Design review of the part built by this model. Coordinates are the model's own, in mm. A direction names the side the tool comes from. Coordinates: 2 decimals unless noted, no trailing zeros. Loops run counter-clockwise (first coordinate to the right, second up) from the corner with the lowest first, then second, coordinate; pieces in that order, holes last.
Autodesk Inventor part; units mm, degrees
ref_plane "YZ Plane" through (0, 0, 0) normal (1, 0, 0) x (0, 1, 0)
ref_plane "XZ Plane" through (0, 0, 0) normal (0, 1, 0) x (-1, 0, 0)
ref_plane "XY Plane" through (0, 0, 0) normal (0, 0, 1) x (1, 0, 0)
sketch "Sketch1" plane through (0, 0, 0) normal (0, 1, 0) x (-1, 0, 0)
  circle A0 centre (0, 0) radius 43.5
  dimension "d0" = 87
extrude "Extrusion1" add sketch "Sketch1" along normal blind 13
sketch "Sketch2" plane through (0, 13, 0) normal (0, 1, 0) x (1, 0, 0)
  circle A0 centre (0, 0) radius 43.5
  line L0 (0, 55.4914) -> (0, 55.5)
  circle A1 centre (0, 0) radius 43.5
  line L1 (43.5, 0) -> (43.5, 37)
  line L2 (0, 55.5) -> (1, 55.5)
  line L3 (1, 55.5) -> (1, 43.5)
  line L4 (0, 55.4914) -> (0, 55.5)
  arc A2 (43.5, 37) -> (1, 55.5) centre (1, -2.5676) ccw
  line L5 (1, 43.4885) -> (1, 43.5)
  line L6 (-55.5, 1) -> (-43.5, 1)
  arc A3 (-37, 43.5) -> (-55.5, 1) centre (2.5676, 1) ccw
  line L7 (0, 43.5) -> (-37, 43.5)
  line L8 (-1, -55.5) -> (-1, -43.5)
  arc A4 (-43.5, -37) -> (-1, -55.5) centre (-1, 2.5676) ccw
  line L9 (-43.5, 0) -> (-43.5, -37)
  line L10 (55.5, -1) -> (43.5, -1)
  arc A5 (37, -43.5) -> (55.5, -1) centre (-2.5676, -1) ccw
  line L11 (0, -43.5) -> (37, -43.5)
  point P0 (0, 43.5)
  point P1 (43.5, 0)
  point P2 (-55.4914, 0)
  point P3 (0, -55.4914)
  point P4 (55.4914, 0)
  dimension "d3" = 12
  dimension "d75" = 1
  dimension "d91" = 37
  dimension "d92" = 58.0676
  dimension "d93" = 42.5
  dimension "d94" = 0
  dimension "d95" = 87.5
  dimension "d110" = 360
extrude "Extrusion2" add sketch "Sketch2" against normal blind 13 contours A0 L5 L3 A2 L1
sketch "Sketch6" plane through (0, 0, 0) normal (0, -1, 0) x (1, 0, 0)
  circle A0 centre (0, 0) radius 43.5
  point P0 (0, 43.5)
sketch "Sketch17" plane through (0, 13, 0) normal (0, 1, 0) x (1, 0, 0)
  circle A0 centre (0, 0) radius 25
  dimension "d141" = 50
extrude "Extrusion16" add sketch "Sketch17" along normal blind 2
sketch "Sketch7" plane through (0, 13, 0) normal (0, 1, 0) x (1, 0, 0)
  circle A0 centre (0, 0) radius 37.5
  dimension "d23" = 75
extrude "Extrusion5" add sketch "Sketch7" along normal blind 15
extrude "Extrusion6" add sketch "Sketch6" along normal blind 79
sketch "Sketch8" plane through (0, -79, 0) normal (0, -1, 0) x (1, 0, 0)
  line L0 (0, -43.5) -> (0, -55.5)
  line L1 (0, -43.4937) -> (0, -55.5)
  line L2 (43.4937, 0) -> (55.5, 0)
  line L3 (0, 43.4937) -> (0, 55.5)
  line L4 (-43.4937, 0) -> (-55.5, 0)
  line L5 (-55.5, -2) -> (-43.5, -2)
  circle A0 centre (0, 0) radius 43.5
  line L6 (-43.5, 0) -> (-55.5, 0)
  line L7 (-55.5, 0) -> (-55.5, -2)
  line L8 (-43.5, 0) -> (-43.5, -37)
  circle A1 centre (0, 0) radius 43.5
  line L9 (-55.5, 0) -> (-55.5, 1)
  line L10 (-55.5, 1) -> (-43.4885, 1)
  line L11 (0, -43.5) -> (37, -43.5)
  line L12 (-1, -55.5) -> (-1, -43.4885)
  line L13 (2, -55.5) -> (2, -43.5)
  line L14 (0, -55.5) -> (2, -55.5)
  line L15 (0, -55.5) -> (-1, -55.5)
  circle A2 centre (0, 0) radius 43.5
  line L16 (43.5, 0) -> (43.5, 37)
  line L17 (55.5, -1) -> (43.4885, -1)
  line L18 (55.5, 2) -> (43.5, 2)
  line L19 (55.5, 0) -> (55.5, 2)
  line L20 (55.5, 0) -> (55.5, -1)
  circle A3 centre (0, 0) radius 43.5
  line L21 (0, 43.5) -> (-37, 43.5)
  line L22 (1, 55.5) -> (1, 43.4885)
  line L23 (-2, 55.5) -> (-2, 43.5)
  line L24 (0, 55.5) -> (-2, 55.5)
  line L25 (0, 55.5) -> (1, 55.5)
  circle A4 centre (0, 0) radius 43.5
  line L26 (-2, -43.5) -> (-37, -43.5)
  arc A5 (-43.5, -37) -> (-1, -55.5) centre (-3.75, -3.75) ccw
  arc A6 (37, -43.5) -> (55.5, -1) centre (3.75, -3.75) ccw
  line L27 (0, -43.5) -> (37, -43.5)
  line L28 (2, -55.5) -> (2, -43.5)
  line L29 (-1, -55.5) -> (-1, -43.4885)
  line L30 (0, -55.5) -> (2, -55.5)
  arc A7 (43.5, 37) -> (1, 55.5) centre (3.75, 3.75) ccw
  line L31 (43.5, 0) -> (43.5, 37)
  line L32 (55.5, 2) -> (43.5, 2)
  line L33 (55.5, -1) -> (43.4885, -1)
  line L34 (55.5, 0) -> (55.5, 2)
  arc A8 (-37, 43.5) -> (-55.5, 1) centre (-3.75, 3.75) ccw
  line L35 (0, 43.5) -> (-37, 43.5)
  line L36 (-2, 55.5) -> (-2, 43.5)
  line L37 (1, 55.5) -> (1, 43.4885)
  line L38 (0, 55.5) -> (-2, 55.5)
  line L39 (-43.5, -37) -> (0, -37)
  line L40 (0, -37) -> (0, -55.5)
  point P0 (43.5, 0)
  point P1 (0, 43.5)
  point P2 (-43.5, 0)
  point P3 (43.5, -37)
  point P4 (37, 43.5)
  point P5 (-43.5, 37)
  point P6 (43.5, 0)
  point P7 (0, 43.5)
  point P8 (-43.5, 0)
  dimension "d30" = 360
  dimension "d32" = 2
  dimension "d33" = 12
  dimension "d52" = 35
  dimension "d60" = 1
  dimension "d67" = 360
  dimension "d71" = 360
  dimension "d137" = 51.823
  dimension "d138" = 3.75
  dimension "d139" = 43.5
  dimension "d140" = 18.5
extrude "Extrusion7" add sketch "Sketch8" along normal blind 13 contours A0 L39 L40 L1 | L1 L40 L39 A0 | A0 L17 A6 L11 | L12 A5 L39 A0 | L39 L8 A0 | A0 L22 A7 L16 | L10 A8 L21 A0
sketch "Sketch9" plane through (0, -92, 0) normal (0, -1, 0) x (1, 0, 0)
  circle A0 centre (0, 0) radius 37.5
extrude "Extrusion8" add sketch "Sketch9" along normal blind 135
sketch "Sketch10" plane through (0, -227, 0) normal (0, -1, 0) x (1, 0, 0)
  line L0 (-25, 25) -> (25, 25)
  line L1 (25, 25) -> (25, -25)
  line L2 (25, -25) -> (-25, -25)
  line L3 (-25, -25) -> (-25, 25)
  point P0 (0, 0)
  point P1 (0, -25)
  dimension "d43" = 25
  dimension "d44" = 50
  dimension "d45" = 50
  dimension "d46" = 25
extrude "Extrusion9" add sketch "Sketch10" along normal blind 40
sketch "Sketch11" plane through (0, -267, 0) normal (0, -1, 0) x (1, 0, 0)
  circle A0 centre (0, 0) radius 9
  dimension "d49" = 18
extrude "Extrusion10" add sketch "Sketch11" along normal blind 30
pattern_circular "Circular Pattern1" count 4 over 360 about axis through (0, -10, 0) along (0, 1, 0) of "Extrusion2"
sketch "Sketch13" plane through (1, 13, -55.5) normal (-1, 0, 0) x (0, 0, 1)
  line L0 (0, 0) -> (0, -13)
  line L1 (0, -6.5) -> (12, -6.5)
  line L2 (12, -13) -> (12, 0)
  circle A0 centre (6, -6.5) radius 2.5
  point P0 (55.5, -13)
extrude "Extrusion12" cut sketch "Sketch13" against normal blind 10
pattern_circular "Circular Pattern2" count 4 over 360 about axis through (0, -10, 0) along (0, 1, 0) of "Extrusion12"
sketch "Sketch14" plane through (43.4885, -79, -1) normal (0, 0, 1) x (1, 0, 0)
  line L0 (12.0115, -13) -> (0, -13)
  line L1 (12.0115, 0) -> (0, 0)
  circle A0 centre (6.0115, -6.5) radius 2.5
  line L2 (0.0115, 0) -> (0.0115, -13)
  point P0 (-43.4885, 79)
  point P1 (6.0057, -13)
  point P2 (0.0115, -6.5)
  dimension "d120" = 5
  dimension "d128" = 6.5
  dimension "d129" = 6
extrude "Extrusion13" cut sketch "Sketch14" against normal blind 10
pattern_circular "Circular Pattern3" count 4 over 360 about axis through (0, -10, 0) along (0, 1, 0) of "Extrusion13"
fillet "Fillet1" radius 2 12 edges at (25, -227, 0) (25, -247, 25) (25, -267, 0) (25, -247, -25) (0, -267, -25) (0, -267, 25) (-25, -267, 0) (0, -227, -25) (-25, -247, -25) (-25, -227, 0) (-25, -247, 25) (0, -227, 25)
sketch "Sketch15" plane through (0, 28, 0) normal (0, 1, 0) x (1, 0, 0)
  circle A0 centre (0, 0) radius 75
  dimension "d131" = 150
extrude "Extrusion14" add sketch "Sketch15" along normal blind 170
sketch "Sketch16" plane through (0, 198, 0) normal (0, 1, 0) x (1, 0, 0)
  circle A0 centre (0, 0) radius 9
  circle A1 centre (0, 0) radius 74
  dimension "d134" = 148
extrude "Extrusion15" cut sketch "Sketch16" against normal blind 120 contours A0 | A1
properties part number "Carbon_Fibre" material "Steel"
Q1. The part is to be moulded in two halves that separate along Z. For faces 1 (the flat face through (40, -79, -25)), 2 (the cylindrical face through (-43.46, -38.76, -1.91)), 3 (the cylindrical face through (-16.04, 138.84, 72.24)), say which applies: pulls with the +Z half, pulls with the -Z half, needs draft (parallel to the pull), parting line crosses it, or undercut.
Q2. Take a section at B-B, the plane z = 65. Write out the cut boundary in (x, y).
Q3. Machinability: for faces 4 (the flat face through (25, -247, 0)), 5 (the flat face through (18, -85, -43.5)), 6 (the flat face through (-43.5, 7, 18)), which of the approach directions +Z, -Z, +X, -X, +Y, -Y give a long, thin tool a straight path to every point of the face, cutting with its end or side? Answer none if there is none.
Q4. Take a section at C-C, the plane y = 57. Write out the cut boundary in (x, z), then the cut area to 3 significant figures.
Q5. Take a section at A-A, the plane y = -253. Write out the cut boundary in (x, z), then the cut area to 3 significant figures.
Q6. Clearance check with flat-ended pins moving along their axes: pin 1 Ø3 at (x, z) = (-18, -39.5) entering from -Y; pin 2 Ø6 at (x, y) = (49.5, -85.5) entering from -Z; pin 3 Ø6 at (y, z) = (-86, -50.5) entering from +X; pin 4 Ø4 at (x, y) = (-40.5, -136) entering from +Z. State where each tip first meets the part, or that it passes through.
Q7. For line 1 (Y direction, x = -7.5, z = 49.5); line 2 (Y direction, x = -49.5, z = 8); line 3 (Y direction, x = -34.5, z = -20.5), list the stretches that pass through material, from the lowest coordinate up.
Entries:
1. face 1: needs draft
1. face 2: parting line crosses it
1. face 3: undercut
2. outline: (-37.42, 28) - (37.42, 28) - (37.42, 198) - (35.37, 198) - (35.37, 78) - (-35.37, 78) - (-35.37, 198) - (-37.42, 198) - close
3. face 4: +Z, -Z, +X, -Y
3. face 5: -Z, +X, -Y
3. face 6: +Z, -X
4. outline: circle Ø150 at (0, 0)
4. area: 17,700 mm2
5. outline: (-25, -23) arc R2 ccw to (-23, -25) - (23, -25) arc R2 ccw to (25, -23) - (25, 23) arc R2 ccw to (23, 25) - (-23, 25) arc R2 ccw to (-25, 23) - close
5. area: 2,500 mm2
6. pin 1: stops at y = -92
6. pin 2: stops at z = -33.04
6. pin 3: stops at x = -1
6. pin 4: passes through
7. line 1: y = 0 to 4, 9 to 13, 28 to 78
7. line 2: y = -92 to -88, -83 to -79, 28 to 78
7. line 3: y = -92 to 13, 28 to 78
